Work out the finished part from the listing and answer in its coordinate system (mm). A direction names the side the tool comes from. Round coordinates to 2 decimals unless told otherwise and drop trailing zeros. Write each loop counter-clockwise with the first axis right and the second up, starting at its lowest first coordinate (ties: lowest second). Pieces come first, ordered by that corner, then holes. Notation, with made-up numbers: (-11.75, 32.25) - (21.25, 32.25) arc R16 ccw to (21.25, 60.25) - close; hole circle Ø10 at (51, 15). An arc over 180 degrees is marked (long way). Answer as a JSON object with one key per item and string values.
```python
from build123d import *

# Parameters (mm, degrees)
SKETCH1_W          = 76.2
SKETCH1_H          = 2.0828
CHAMFER1_SIZE      = 0.5953125
SKETCH4_R          = 3.9624
EXTRUDE1_DEPTH     = 2.2098
CUT_EXTRUDE1_DEPTH = 1.1049
SKETCH7_R          = 1.374815329
CUT_EXTRUDE4_DEPTH = 1.1049
CUT_EXTRUDE4_TAPER = 45
SKETCH8_R          = 1.190625
CUT_EXTRUDE5_DEPTH = 0.3683
CUT_EXTRUDE5_TAPER = 60


with BuildPart() as part:
    # Sketch1 → Revolve1 (revolve)
    with BuildSketch(Plane(origin=(0, 0, 0), x_dir=(0, 0, -1), z_dir=(1, 0, 0))):
        with Locations((38.1, 1.0414)):
            Rectangle(SKETCH1_W, SKETCH1_H)
    revolve(axis=Axis((0, 0, 0), (0, 0, 1)))

    # Chamfer1
    chamfer1_edges = [part.edges().sort_by_distance(p)[0] for p in [
        (0, -2.0828, -76.2),
    ]]
    chamfer(chamfer1_edges, length=CHAMFER1_SIZE)

    # Sketch4 → Extrude1 (add)
    with BuildSketch(Plane.XY):
        Circle(SKETCH4_R)
    extrude(amount=EXTRUDE1_DEPTH)

    # Sketch9 → Cut-Revolve3 (revolve, cut)
    with BuildSketch(Plane(origin=(0, 0, 0), x_dir=(0, 0, -1), z_dir=(1, 0, 0))):
        with BuildLine():
            Line((0, 3.9624), (-0.381, 3.9624))
            ThreePointArc((-0.381, 3.9624), (-1.434442989, 3.157885071), (-2.2098, 2.0828))
            Line((-2.2098, 2.0828), (-2.5908, 2.0828))
            Line((-2.5908, 2.0828), (-2.5908, 4.3434))
            Line((-2.5908, 4.3434), (0, 4.3434))
            Line((0, 4.3434), (0, 3.9624))
        make_face()
    revolve(axis=Axis((0, 0, 0), (0, 0, 1)), mode=Mode.SUBTRACT)

    # Sketch6 → Cut-Extrude1 (cut)
    with BuildSketch(Plane.XY.offset(2.2098)):
        Polygon((0, -1.374815329), (1.190625, -0.687407664), (1.190625, 0.687407664), (0, 1.374815329), (-1.190625, 0.687407664), (-1.190625, -0.687407664), align=None)
    extrude(amount=-CUT_EXTRUDE1_DEPTH, mode=Mode.SUBTRACT)

    # Sketch7 → Cut-Extrude4 (cut)
    with BuildSketch(Plane.XY.offset(2.2098)):
        Circle(SKETCH7_R)
    extrude(amount=-CUT_EXTRUDE4_DEPTH, taper=CUT_EXTRUDE4_TAPER, mode=Mode.SUBTRACT)

    # Sketch8 → Cut-Extrude5 (cut)
    with BuildSketch(Plane.XY.offset(1.1049)):
        Circle(SKETCH8_R)
    extrude(amount=-CUT_EXTRUDE5_DEPTH, taper=CUT_EXTRUDE5_TAPER, mode=Mode.SUBTRACT)


solid = part.part
```
Item 1: A cutting plane is placed at A-A (z = -35). Write down the section's boundary in (x, y), and give its area (3 significant figures).
Results found:
{"outline": "circle Ø4.17 at (0, 0)", "area": "13.6 mm²"}
Item 2: Consider line 1 along Z through (x, y) = (2.25, -3); line 2 along Z through (x, y) = (2, 2.5); line 3 along X through (y, z) = (-1.25, -4). Determine where each line is inside the solid, lowest interval first.
Results found:
{"line 1": "0 to 0.73", "line 2": "0 to 1.39", "line 3": "-1.67 to 1.67"}
Item 3: Each of these flat-tipped pins is pushed along its axis until it touches: P1, Ø0.9, axis at y = 0, z = 2, coming from the -X side; P2, Ø1.5, axis at y = 2, z = -12, coming from the -X side; P3, Ø0.7, axis at x = -1, y = 0.5, coming from the +Z side; P4, Ø1, axis at x = 2, z = -8, coming from the +Y side (3 decimals). Where does it stop, or does it pass through?
Results found:
{"P1": "x = -3.03", "P2": "x = -1.67", "P3": "z = 2.21", "P4": "y = 1.445"}
Item 4: For faces 1 (the cylindrical face through (-0.626, 1.987, -38.332)), 2 (the cylindrical face through (3.66, -1.52, 0.19)), determine the directions among +Z, -Z, +X, -X, +Y, -Y from which every point of the face is accessible in a straight line to the end or side of a thin tool.
Results found:
{"face 1": "-Z", "face 2": "+Z, -Z"}
Item 5: A cutting plane is placed at B-B (x = -2.75). Write down the section's boundary in (y, z), and give its area (3 significant figures).
Results found:
{"outline": "(-2.85, 0) - (2.85, 0) - (2.85, 0.38) arc R3.6 ccw to (-2.85, 0.38) - close", "area": "7.77 mm²"}
